Build history of the part. All positions in model axes, mm. Coordinates: 2 decimals unless noted, no trailing zeros. Order: outer loops, then holes, each group sorted by start corner. A loop starts at its lowest first (then second) coordinate and runs counter-clockwise, first axis right, second up. Notation, with made-up numbers: (67.25, 9.5) - (96.25, 9.5) arc R25 ccw to (96.25, 25.5) - close; hole circle Ø1 at (65.5, 66.25). An arc over 180 degrees is marked (long way). Answer as CSV lines item,"result". Start each with the question number.
from build123d import *

# Parameters (mm, degrees)
SKETCH_1_R      = 7.75
SKETCH_1_R_2    = 2.1
EXTRUDE_1_DEPTH = 5


with BuildPart() as part:
    # 草图1 → 凸台-拉伸1 (new body)
    with BuildSketch(Plane(origin=(0, 0, 0), x_dir=(1, 0, 0), z_dir=(0, 1, 0))):
        with BuildLine():
            Line((15, 0), (15, 35))
            ThreePointArc((15, 35), (0, 50), (-15, 35))
            Line((-15, 35), (-15, 0))
            Line((-15, 0), (15, 0))
        make_face()
        with Locations(Location((0, 35, 0), (0, 0, 270))):
            Circle(SKETCH_1_R, mode=Mode.SUBTRACT)
        with Locations(Location((-6, 5.5, 0), (0, 0, 270))):
            Circle(SKETCH_1_R_2, mode=Mode.SUBTRACT)
        with Locations(Location((6, 5.5, 0), (0, 0, 270))):
            Circle(SKETCH_1_R_2, mode=Mode.SUBTRACT)
    extrude(amount=EXTRUDE_1_DEPTH)


solid = part.part
(1) Drop flat-ended pins along their axis: pin 1 Ø2 at (x, y) = (7, 1.5) entering from -Z; pin 2 Ø4 at (x, z) = (6, -5.5) entering from -Y. Give the stop position or say it passes through.
(2) Band-saw the part on D-D on x = 6. List the corners of the cut face in (y, z), plus the area to 3 significant figures.
(3) Probe L1, parallel to X at y = 1.1, z = -5.5; L2, parallel to X at y = 3.4, z = -4.5; L3, parallel to X at y = 1.25, z = -37. List the from-to ranges inside material, lowest first. Write a range as [from, to].
(4) Band-saw the part on A-A on y = 3.4. List the corners of the cut face in (x, z), plus the area to 3 significant figures.
(5) Pull direction X, two halves, no side cores. Call faces 1 (the flat face through (15, 2, -17)), 2 (the flat face through (0, 2, 0)), 3 (the cylindrical face through (-7.863, 2.465, -4.531)): +X half, -X half, draft (parallel to the pull), parting line (faces both ways), or undercut.
(6) Band-saw the part on B-B on z = -5.5. List the corners of the cut face in (x, y).
(7) Band-saw the part on C-C on x = 0. List the corners of the cut face in (y, z), plus the area to 4 significant figures.
Filled in:
1,pin 1,"stops at z = -48.75"
1,pin 2,"passes through"
2,outline,"(0, -48.75) - (5, -48.75) - (5, -39.91) - (0, -39.91) - close; (0, -30.09) - (5, -30.09) - (5, -7.6) - (0, -7.6) - close; (0, -3.4) - (5, -3.4) - (5, 0) - (0, 0) - close"
2,area,"174 mm^2"
3,L1,"x = [-15, -8.1], [-3.9, 3.9], [8.1, 15]"
3,L2,"x = [-15, -7.85], [-4.15, 4.15], [7.85, 15]"
3,L3,"x = [-14.87, -7.49], [7.49, 14.87]"
4,outline,"(-15, -35) arc R15 ccw to (15, -35) - (15, 0) - (-15, 0) - close; hole circle Ø4.2 at (-6, -5.5); hole circle Ø15.5 at (0, -35); hole circle Ø4.2 at (6, -5.5)"
4,area,"1,190 mm^2"
5,face 1,"+X half"
5,face 2,"draft"
5,face 3,"undercut"
6,outline,"(-15, 0) - (-8.1, 0) - (-8.1, 5) - (-15, 5) - close; (-3.9, 0) - (3.9, 0) - (3.9, 5) - (-3.9, 5) - close; (8.1, 0) - (15, 0) - (15, 5) - (8.1, 5) - close"
7,outline,"(0, -50) - (5, -50) - (5, -42.75) - (0, -42.75) - close; (0, -27.25) - (5, -27.25) - (5, 0) - (0, 0) - close"
7,area,"172.5 mm^2"
